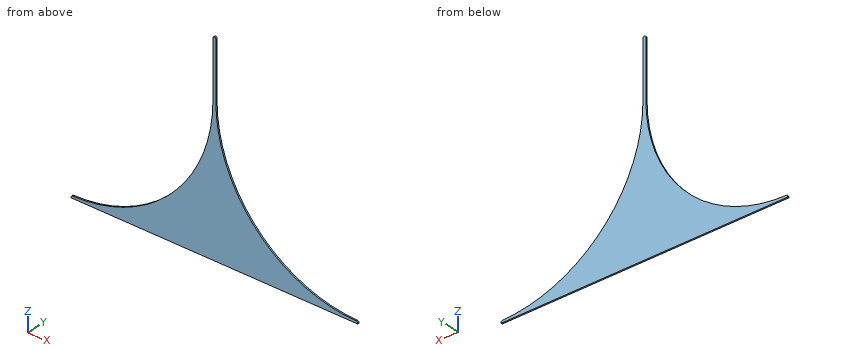
from build123d import *

# Parameters (mm, degrees)
BASE_FLANGE1_DEPTH = 2


# Sheet-metal steps are written as plain solids
with BuildPart() as part:
    # Sketch1 → Base-Flange1 (new body)
    with BuildSketch(Plane(origin=(0, 0, 0), x_dir=(1, 0, 0), z_dir=(0, 1, 0))):
        with BuildLine():
            Line((0, 0), (398, 0))
            Line((398, 0), (398, -1.109075119))
            ThreePointArc((398, -1.109075119), (397.449904564, -2.446145673), (396.118149824, -3.008988429))
            ThreePointArc((396.118149824, -3.008988429), (258.03621096, -61.36689516), (201, -200))
            Line((201, -200), (201, -278.1))
            ThreePointArc((201, -278.1), (200.443502884, -279.443502884), (199.1, -280))
            Line((199.1, -280), (199, -280))
            Line((199, -280), (198.9, -280))
            ThreePointArc((198.9, -280), (197.556497116, -279.443502884), (197, -278.1))
            Line((197, -278.1), (197, -200))
            ThreePointArc((197, -200), (139.96378904, -61.36689516), (1.881850176, -3.008988429))
            ThreePointArc((1.881850176, -3.008988429), (0.550095436, -2.446145673), (0, -1.109075119))
            Line((0, -1.109075119), (0, 0))
        make_face()
    extrude(amount=-BASE_FLANGE1_DEPTH)


solid = part.part
Design review of the part built by this model. Coordinates are the model's own, in mm. Give positions to 0.01 mm unless a question says otherwise; leave off trailing zeros. Order: outer loops, then holes, each group sorted by start corner. A loop starts at its lowest first (then second) coordinate and runs counter-clockwise, first axis right, second up. Notation, with made-up numbers: (8.25, -19) - (15.25, -19) arc R31 ccw to (15.25, 7) - close; hole circle Ø1 at (-10.75, -9). An arc over 180 degrees is marked (long way). Write item = value, one per line. Start each with the question number.
Q1. We need section C-C on x = 304.5. State the section outline as (y, z) points, plus the area to 3 significant figures.
Q2. Clearance check with flat-ended pins moving along their axes: pin 1 Ø0.6 at (y, z) = (-1.5, 228) entering from +X; pin 2 Ø1 at (x, y) = (42.5, -0.5) entering from +Z. State where each tip first meets the part, or that it passes through.
Q3. To check wall thickness, follow L1, parallel to X at y = -1.6, z = 251; L2, parallel to Z at x = 200, y = -1.5; L3, parallel to Z at x = 297, y = -1.7. State the ranges of each line that lie inside material, in increasing order. Write a range as from..to.
Q4. We need section B-B on z = 224.5. State the section outline as (x, y) points, plus the area to 3 significant figures.
Q5. We need section A-A on y = -1.4. State the section outline as (x, z) points.
Working result:
q1.outline = (-2, 0) - (0, 0) - (0, 26.6) - (-2, 26.6) - close
q1.area = 53.2 mm²
q2.pin_1 = 201
q2.pin_2 = 7.75
q3.L1 = 197..201
q3.L2 = 0..279.77
q3.L3 = 0..30.86
q4.outline = (197, -2) - (201, -2) - (201, 0) - (197, 0) - close
q4.area = 8.00 mm²
q5.outline = (0, 0) - (398, 0) - (398, 1.11) arc R1.9 ccw to (396.12, 3.01) arc R197 cw to (201, 200) - (201, 278.1) arc R1.9 ccw to (199.1, 280) - (198.9, 280) arc R1.9 ccw to (197, 278.1) - (197, 200) arc R197 cw to (1.88, 3.01) arc R1.9 ccw to (0, 1.11) - close
